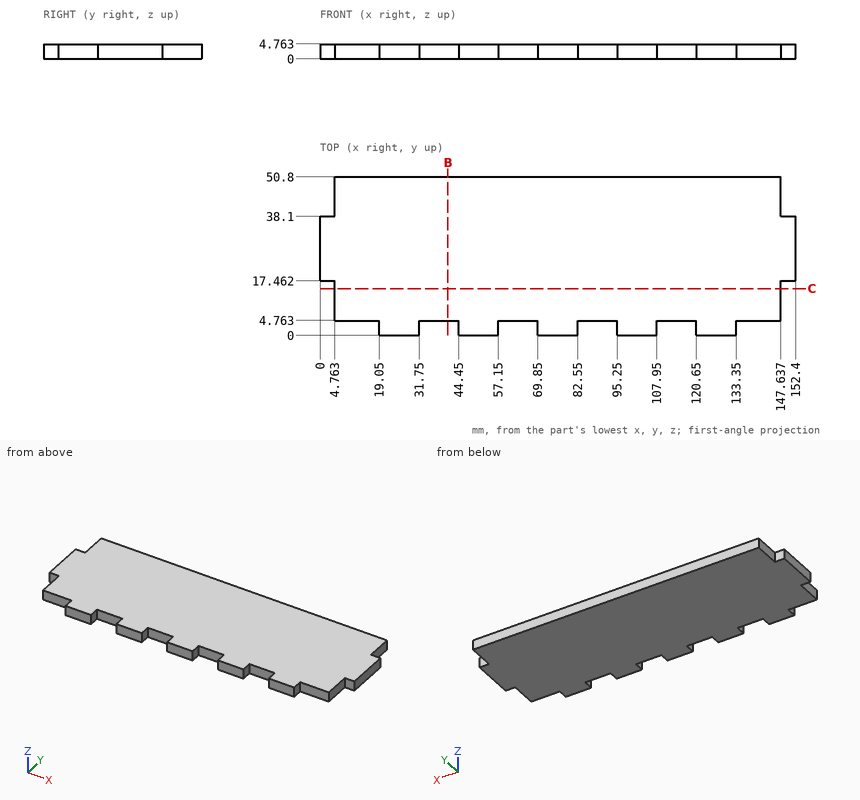
Verification items for this drawing (mm, ordinates from the low corner). Give positions to 0.01 mm unless a question says otherwise; leave off trailing zeros. Loops run counter-clockwise (first coordinate to the right, second up) from the corner with the lowest first, then second, coordinate; pieces in that order, holes last.
1. Cross-section at C-C on y = 15. Record the cut outline in (x, z).
Derived:
outline: (4.76, 0) - (147.64, 0) - (147.64, 4.76) - (4.76, 4.76) - close
2. Cross-section at B-B on x = 41. Record the cut outline in (y, z).
Derived:
outline: (4.76, 0) - (50.8, 0) - (50.8, 4.76) - (4.76, 4.76) - close
3. Material ranges on probe 1 along X at (y, z) = (4, 4.2); probe 2 along Y at (x, z) = (115.5, 0.5); probe 3 along X at (y, z) = (9.5, 0.6), recorded low to high.
Derived:
probe 1: x = 19.05 to 31.75, 44.45 to 57.15, 69.85 to 82.55, 95.25 to 107.95, 120.65 to 133.35
probe 2: y = 4.76 to 50.8
probe 3: x = 4.76 to 147.64
4. Go/stop test with flat-tipped pins: P1, Ø1.4, axis at x = 11, z = 2, coming from the -Y side; P2, Ø2.5, axis at x = 149, z = 3, coming from the -Y side; P3, Ø1.5, axis at y = 13, z = 4.5, coming from the +X side. Record where each tip stops, or that it passes through.
Derived:
P1: stops at y = 4.76
P2: stops at y = 17.46
P3: stops at x = 147.64
